from build123d import *

# Parameters (mm, degrees)
SKETCH_3_R               = 1.5
CUT_EXTRUDE_2_DEPTH      = 119.764820154
PATTERN_CIRCULAR_2_COUNT = 3
SKETCH_4_W               = 24
SKETCH_4_H               = 40
SKETCH_4_W_2             = 13
SKETCH_4_H_2             = 23
EXTRUDE_1_DEPTH          = 6
EXTRUDE_2_REACH          = 122.983
SKETCH_5_W               = 24
SKETCH_5_H               = 5.196152423
EXTRUDE_3_REACH          = 166.046
EXTRUDE_3_END_RADIUS     = 74
SKETCH_8_W               = 24
SKETCH_8_H               = 11.158003069


with BuildPart() as part:
    # Sketch 1 → Revolve 1 (revolve)
    with BuildSketch(Plane.XY):
        with BuildLine():
            Line((19.152609338, 71.478511145), (0, 71.478511145))
            Line((0, 71.478511145), (0, 67.478511145))
            Line((0, 67.478511145), (18.618553478, 67.478511145))
            ThreePointArc((18.618553478, 67.478511145), (45.193772934, 53.455803127), (63.441545093, 29.583278322))
            Line((63.441545093, 29.583278322), (67.066776241, 31.273751369))
            ThreePointArc((67.066776241, 31.273751369), (47.566283117, 56.687288791), (19.152609338, 71.478511145))
        make_face()
    revolve(axis=Axis((0, 0, 0), (0, 1, 0)))

    # Sketch 3 → Cut-Extrude 2 (cut, through all)
    with BuildSketch(Plane(origin=(0, 0, 0), x_dir=(-1, 0, 0), z_dir=(0, 0.500000000000001, 0.866025403784438))):
        with Locations(Location((0, 0, 0), (0, 0, 270))):
            Circle(SKETCH_3_R)
    cut_extrude_2 = extrude(amount=CUT_EXTRUDE_2_DEPTH, mode=Mode.SUBTRACT)

    # Pattern Circular 2: Cut-Extrude 2 ×3 about axis
    pattern_circular_2_axis = Axis((0, 71.478511145, 0), (0, -1, 0))
    for i in range(1, PATTERN_CIRCULAR_2_COUNT):
        add(cut_extrude_2.rotate(pattern_circular_2_axis, i * 360 / PATTERN_CIRCULAR_2_COUNT), mode=Mode.SUBTRACT)



with BuildPart() as body_2:
    # Sketch 4 → Extrude 1 (new body)
    with BuildSketch(Plane(origin=(0, 43, 74.478184725), x_dir=(-1, 0, 0), z_dir=(0, 0.500000000000001, 0.866025403784438))):
        Rectangle(SKETCH_4_W, SKETCH_4_H)
        Rectangle(SKETCH_4_W_2, SKETCH_4_H_2, mode=Mode.SUBTRACT)
    extrude(amount=EXTRUDE_1_DEPTH)

    # Sketch 5 → Extrude 2 (add, up to next)
    with BuildSketch(Plane(origin=(0, 71.478511145, 0), x_dir=(1, 0, 0), z_dir=(0, 1, 0)), mode=Mode.PRIVATE) as extrude_2_sk1:
        with Locations((0, -67.076260937)):
            Rectangle(SKETCH_5_W, SKETCH_5_H)
    extrude_2_tool1 = extrude(extrude_2_sk1.sketch, amount=-EXTRUDE_2_REACH, mode=Mode.PRIVATE) - body_2.part
    add(extrude_2_tool1.solids().sort_by_distance((0, 71.478511, 67.076261))[0])


with BuildPart() as part_1:
    add(part.part)

    add(body_2.part)  # Extrude 3 merges body 2
    # Extrude 3: up to this sphere (the profile starts outside it)
    extrude_3_end = Location((0, 0, 0)) * Sphere(EXTRUDE_3_END_RADIUS, mode=Mode.PRIVATE)
    # Sketch 8 → Extrude 3 (add, up to the surface)
    with BuildSketch(Plane(origin=(0, 0, 64.478184725), x_dir=(-1, 0, 0), z_dir=(0, 0, -1)), mode=Mode.PRIVATE) as extrude_3_sk1:
        with Locations((0, 65.899509611)):
            Rectangle(SKETCH_8_W, SKETCH_8_H)
    extrude_3_tool1 = extrude(extrude_3_sk1.sketch, amount=EXTRUDE_3_REACH, mode=Mode.PRIVATE) - extrude_3_end
    add(extrude_3_tool1.solids().sort_by_distance((0, 65.89951, 64.478185))[0])


solid = part_1.part
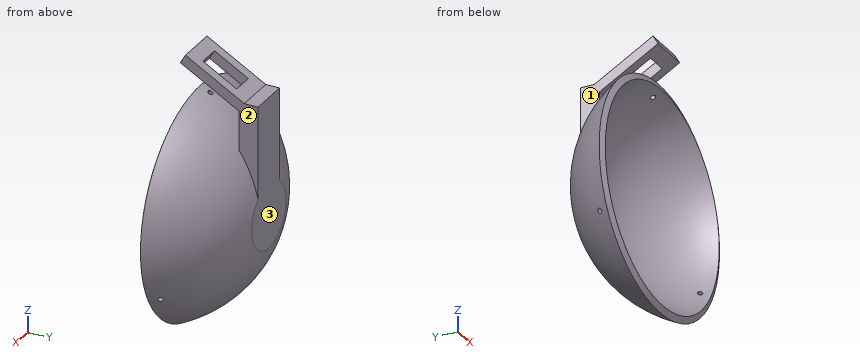
Here's how the part is built. I have some questions about the finished solid (model axes, mm). Face numbers are marked on the shaded views. A direction names the side the tool comes from. Coordinates: 2 decimals unless noted, no trailing zeros. Loops run counter-clockwise (first coordinate to the right, second up) from the corner with the lowest first, then second, coordinate; pieces in that order, holes last.
1. Imagine slicing it at B-B, the plane z = 0. Please give me the cut outline in (x, y), and give its area (3 significant figures).
2. Imagine slicing it at A-A, the plane y = 48. Please give me the cut outline in (x, z), and give its area (3 significant figures).
3. I need wall thicknesses on L1, parallel to Z at x = 1.5, y = 54; L2, parallel to Z at x = -18.5, y = 51; L3, parallel to Z at x = -13, y = 45.5. Which ranges of each line are inside material? Lowest first, please.
4. For P1, Ø6, axis at x = -8, y = 42, coming from the -Z side; P2, Ø7, axis at x = -2.5, z = 53, coming from the -Y side; P3, Ø13.5, axis at y = 37.5, z = 61, coming from the +X side (3 decimals), each with a flat end and sliding along its axis, tell me the tip position at first contact or that it passes through.
5. For the marked faces 1, 2 and 3, which set-ups out of +Z, -Z, +X, -X, +Y, -Y let a thin tool reach every point of the face, with its end or its side?
Taken from the geometry:
1. outline: (-67.07, 31.27) - (-63.44, 29.58) arc R70 cw to (-18.62, 67.48) - (18.62, 67.48) arc R70 cw to (63.44, 29.58) - (67.07, 31.27) arc R74 ccw to (19.15, 71.48) - (-19.15, 71.48) arc R74 ccw to start
1. area: 652 mm2
2. outline: circle Ø112.64 at (0, 0); (-12, 71.59) - (-6.5, 71.59) - (-6.5, 78.52) - (-12, 78.52) - close; (6.5, 71.59) - (12, 71.59) - (12, 78.52) - (6.5, 78.52) - close; hole circle Ø101.9 at (0, 0)
2. area: 1,890 mm2
3. L1: z = -50.57 to -44.52, 44.52 to 50.57, 68.13 to 70.53
3. L2: z = -50.33 to -44.24, 44.24 to 50.33
3. L3: z = -56.89 to -51.58, 51.58 to 56.89
4. P1: stops at z = -62.41
4. P2: stops at y = 41.24
4. P3: stops at x = 35.635
5. face 1: +Z, -X, +Y
5. face 2: +Z, +X, +Y
5. face 3: +Z, -Z, +X, -X, +Y
